from build123d import *

# Parameters (mm, degrees)
F1_DEPTH       = 6
F3_DEPTH       = 25
F4_R           = 30
F4_R_2         = 18.6
F5_DEPTH       = 30
F6_R           = 18.5
F7_DEPTH       = 25
F9_DEPTH       = 25
F9_DEPTH_BACK  = 25
F11_DEPTH      = 25
F11_DEPTH_BACK = 25
F13_DEPTH      = 60.001
F13_DEPTH_BACK = 85.001
F14_R          = 2.6
F15_DEPTH      = 82.066510674
F15_DEPTH_BACK = 82.066510674


with BuildPart() as f1:
    # F0 (on Top) → F1 (new body)
    with BuildSketch(Plane.XY):
        with BuildLine():
            ThreePointArc((82.1416340365, -21.8575377801), (84.2823792174, -11.0218216937), (85, 0))
            ThreePointArc((85, 0), (84.2823792174, 11.0218216937), (82.1416340365, 21.8575377801))
            Line((82.1416340365, 21.8575377801), (-22.1416340365, 82.065510674))
            ThreePointArc((-22.1416340365, 82.065510674), (-42.5, 73.6121593217), (-60, 60.207972894))
            Line((-60, 60.207972894), (-60, -60.207972894))
            ThreePointArc((-60, -60.207972894), (-42.5, -73.6121593217), (-22.1416340365, -82.065510674))
            Line((-22.1416340365, -82.065510674), (82.1416340365, -21.8575377801))
        make_face()
    extrude(amount=F1_DEPTH)

    # F2 (on face) → F3 (cut)
    with BuildSketch(Plane.XY.offset(6)):
        with BuildLine():
            ThreePointArc((71.454527972, -2.5495945353), (71.4886310891, -1.275), (71.5, 0))
            ThreePointArc((71.5, 0), (71.4886310891, 1.275), (71.454527972, 2.5495945353))
            ThreePointArc((71.454527972, 2.5495945353), (68.95, 0), (71.454527972, -2.5495945353))
        make_face()
        with BuildLine():
            ThreePointArc((71.454527972, 2.5495945353), (71.4886310891, 1.275), (71.5, 0))
            ThreePointArc((71.5, 0), (71.4886310891, -1.275), (71.454527972, -2.5495945353))
            ThreePointArc((71.454527972, -2.5495945353), (73.2869731851, -1.8191280427), (74.05, 0))
            ThreePointArc((74.05, 0), (73.2869731851, 1.8191280427), (71.454527972, 2.5495945353))
        make_face()
        with BuildLine():
            ThreePointArc((-37.935277623, -60.6066391715), (-37.025, -64.1291811502), (-33.5192503491, -63.1562337069))
            ThreePointArc((-33.5192503491, -63.1562337069), (-35.75, -61.9208163706), (-37.935277623, -60.6066391715))
        make_face()
        with BuildLine():
            ThreePointArc((-37.935277623, -60.6066391715), (-35.75, -61.9208163706), (-33.5192503491, -63.1562337069))
            ThreePointArc((-33.5192503491, -63.1562337069), (-33.2811023097, -62.5588165234), (-33.2, -61.9208163706))
            ThreePointArc((-33.2, -61.9208163706), (-35.0680754949, -59.4636881751), (-37.935277623, -60.6066391715))
        make_face()
        with BuildLine():
            ThreePointArc((-37.935277623, 60.6066391715), (-35.75, 61.9208163706), (-33.5192503491, 63.1562337069))
            ThreePointArc((-33.5192503491, 63.1562337069), (-37.025, 64.1291811502), (-37.935277623, 60.6066391715))
        make_face()
        with BuildLine():
            ThreePointArc((-33.2, 61.9208163706), (-33.2811023097, 62.5588165234), (-33.5192503491, 63.1562337069))
            ThreePointArc((-33.5192503491, 63.1562337069), (-35.75, 61.9208163706), (-37.935277623, 60.6066391715))
            ThreePointArc((-37.935277623, 60.6066391715), (-35.0680754949, 59.4636881751), (-33.2, 61.9208163706))
        make_face()
    extrude(amount=-F3_DEPTH, mode=Mode.SUBTRACT)

    # F4 (on face) → F5 (join)
    with BuildSketch(Plane.XY.offset(6)):
        Circle(F4_R)
        Circle(F4_R_2, mode=Mode.SUBTRACT)
    extrude(amount=F5_DEPTH)

    # F6 (on face) → F7 (cut)
    with BuildSketch(Plane.XY.offset(6)):
        Circle(F6_R)
    extrude(amount=-F7_DEPTH, mode=Mode.SUBTRACT)

    # F8 (on Right) → F9 (cut, two sides)
    with BuildSketch(Plane.YZ) as f9_sk:
        Polygon((-2.3094010768, 11), (2.3094010768, 11), (4.6188021535, 15), (2.3094010768, 19), (-2.3094010768, 19), (-4.6188021535, 15), align=None)
    extrude(amount=F9_DEPTH, mode=Mode.SUBTRACT)
    extrude(f9_sk.sketch, amount=-F9_DEPTH_BACK, mode=Mode.SUBTRACT)

    # F10 (on Front) → F11 (cut, two sides)
    with BuildSketch(Plane.XZ) as f11_sk:
        Polygon((-2.3094010768, 11), (2.3094010768, 11), (4.6188021535, 15), (2.3094010768, 19), (-2.3094010768, 19), (-4.6188021535, 15), align=None)
    extrude(amount=F11_DEPTH, mode=Mode.SUBTRACT)
    extrude(f11_sk.sketch, amount=-F11_DEPTH_BACK, mode=Mode.SUBTRACT)

    # F12 (on Right) → F13 (cut, two sides)
    with BuildSketch(Plane.YZ) as f13_sk:
        with BuildLine():
            ThreePointArc((0, 17.6), (-2.6, 15), (0, 12.4))
            Line((0, 12.4), (0, 17.6))
        make_face()
        with BuildLine():
            Line((0, 17.6), (0, 12.4))
            ThreePointArc((0, 12.4), (1.8384776311, 13.1615223689), (2.6, 15))
            ThreePointArc((2.6, 15), (1.8384776311, 16.8384776311), (0, 17.6))
        make_face()
    extrude(amount=-F13_DEPTH, mode=Mode.SUBTRACT)
    extrude(f13_sk.sketch, amount=F13_DEPTH_BACK, mode=Mode.SUBTRACT)

    # F14 (on Front) → F15 (cut, two sides)
    with BuildSketch(Plane.XZ) as f15_sk:
        with Locations((0, 15)):
            Circle(F14_R)
    extrude(amount=F15_DEPTH, mode=Mode.SUBTRACT)
    extrude(f15_sk.sketch, amount=-F15_DEPTH_BACK, mode=Mode.SUBTRACT)


solid = f1.part
Geometry: final body of the model. Coordinates: model frame, mm. A direction names the side the tool comes from. Coordinates: 2 decimals unless noted, no trailing zeros. Order: outer loops, then holes, each group sorted by start corner. A loop starts at its lowest first (then second) coordinate and runs counter-clockwise, first axis right, second up.
1) Draft query along X for faces 1 (the flat face through (28, -17, 6)), 2 (the flat face through (-25, 2, 17)), 3 (the flat face through (29.27, -52.383, 2.958)). Return one class per face: released by +X, released by -X, zero draft, split by the parting line, or undercut.
Result sheet:
face 1: zero draft
face 2: undercut
face 3: released by +X
2) Set-up query: faces 4 (the cylindrical face through (27.712, -11.49, 20.79)), 5 (the flat face through (-3.448, -21.46, 17.028)), 6 (the cylindrical face through (-0.56, -27.46, 12.46)). Return all of +Z, -Z, +X, -X, +Y, -Y with unobstructed straight access to the full face (end or side cutting, diameter ignored); none if empty.
Result sheet:
face 4: +Z
face 5: none
face 6: +Y, -Y
3) Section C-C (z = 22.5). Return loops of the section in (x, y).
Result sheet:
outline: circle Ø60 at (0, 0); hole circle Ø37.2 at (0, 0)
4) Section B-B (x = -10.5). Return loops of the section in (y, z), then the cut area to 3 significant figures.
Result sheet:
outline: (-75.34, 0) - (-15.23, 0) - (-15.23, 6) - (-15.35, 6) - (-15.35, 36) - (-28.1, 36) - (-28.1, 6) - (-75.34, 6) - close; (15.23, 0) - (75.34, 0) - (75.34, 6) - (28.1, 6) - (28.1, 36) - (15.35, 36) - (15.35, 6) - (15.23, 6) - close
area: 1,490 mm2
5) First-contact query: P1, Ø3, axis at x = 47, y = -17, coming from the +Z side; P2, Ø6.5, axis at y = 2.5, z = 16.5, coming from the -X side; P3, Ø6.5, axis at y = 1, z = 13.5, coming from the +X side. Flat tips, straight axial feed; report the tip coordinate or a pass-through.
Result sheet:
P1: stops at z = 6
P2: stops at x = -30
P3: stops at x = 30
6) Ray query, probe 1 along Z at (x, y) = (0, 27.8); probe 2 along Y at (x, z) = (0, 22.25); probe 3 along Z at (x, y) = (-38.5, 4). Return the intervals inside material, ascending.
Result sheet:
probe 1: z = 0 to 12.4, 17.6 to 36
probe 2: y = -30 to -18.6, 18.6 to 30
probe 3: z = 0 to 6
7) Section A-A (z = 2). Return loops of the section in (x, y), then the cut area to 3 significant figures.
Result sheet:
outline: (-60, -60.21) arc R85 ccw to (-22.14, -82.07) - (82.14, -21.86) arc R85 ccw to (82.14, 21.86) - (-22.14, 82.07) arc R85 ccw to (-60, 60.21) - close; hole circle Ø5.1 at (-35.75, -61.92); hole circle Ø5.1 at (-35.75, 61.92); hole circle Ø37 at (0, 0); hole circle Ø5.1 at (71.5, 0)
area: 15,300 mm2
8) Section D-D (x = -35.75). Return loops of the section in (y, z).
Result sheet:
outline: (-77.12, 0) - (-64.47, 0) - (-64.47, 6) - (-77.12, 6) - close; (-59.37, 0) - (59.37, 0) - (59.37, 6) - (-59.37, 6) - close; (64.47, 0) - (77.12, 0) - (77.12, 6) - (64.47, 6) - close
